```python
from build123d import *

# Parameters (mm, degrees)
SKETCH3_W                                      = 100
SKETCH3_H                                      = 100
BOSS_EXTRUDE2_DEPTH                            = 8
CBORE_FOR_2_SOCKET_HEAD_CAP_SCREW1_D           = 2.4384
CBORE_FOR_2_SOCKET_HEAD_CAP_SCREW1_CBORE_D     = 4.7625
CBORE_FOR_2_SOCKET_HEAD_CAP_SCREW1_CBORE_DEPTH = 2.1844
FILLET1_R                                      = 1
FILLET2_R                                      = 3
FILLET3_R                                      = 3


with BuildPart() as part:
    # Sketch3 → Boss-Extrude2 (new body)
    with BuildSketch(Plane(origin=(0, 0, 0), x_dir=(1, 0, 0), z_dir=(0, 1, 0))):
        Rectangle(SKETCH3_W, SKETCH3_H)
    extrude(amount=BOSS_EXTRUDE2_DEPTH)

    # CBORE for #2 Socket Head Cap Screw1 (through all)
    with Locations(Plane(origin=(-46, 8, 32), x_dir=(0, 0, 1), z_dir=(0, 1, 0))):
        with Locations((0, 0), (14, 14), (-64, 0), (-78, 14.320192801), (-78, 78), (-64, 92), (14, 78), (0, 92)):
            CounterBoreHole(CBORE_FOR_2_SOCKET_HEAD_CAP_SCREW1_D / 2, CBORE_FOR_2_SOCKET_HEAD_CAP_SCREW1_CBORE_D / 2, CBORE_FOR_2_SOCKET_HEAD_CAP_SCREW1_CBORE_DEPTH)

    # Fillet1
    fillet1_edges = [part.edges().sort_by_distance(p)[0] for p in [
        (-50, 8, 0),
        (0, 8, 50),
        (50, 8, 0),
        (0, 8, -50),
    ]]
    fillet(fillet1_edges, radius=FILLET1_R)

    # Fillet2
    # the kernel refuses this fillet: 3 mm, written as the material it takes off along each edge
    with BuildSketch(Plane(origin=(-47, 8, -47), x_dir=(0, 0, -1), z_dir=(1, 0, 0))) as fillet2_piece_1:
        with BuildLine():
            CenterArc((2, -1), 1, 0, 90)
            Line((3, -1), (3, 0))
            Line((3, 0), (2, 0))
        make_face()
    revolve(axis=Axis((-47, 8, -47), (0, 1, 0)), revolution_arc=90, mode=Mode.SUBTRACT)
    with BuildSketch(Plane(origin=(47, 8, -47), x_dir=(1, 0, 0), z_dir=(0, 0, 1))) as fillet2_piece_2:
        with BuildLine():
            CenterArc((2, -1), 1, 0, 90)
            Line((3, -1), (3, 0))
            Line((3, 0), (2, 0))
        make_face()
    revolve(axis=Axis((47, 8, -47), (0, 1, 0)), revolution_arc=90, mode=Mode.SUBTRACT)
    with BuildSketch(Plane(origin=(-47, 8, 47), x_dir=(-1, 0, 0), z_dir=(0, 0, -1))) as fillet2_piece_3:
        with BuildLine():
            CenterArc((2, -1), 1, 0, 90)
            Line((3, -1), (3, 0))
            Line((3, 0), (2, 0))
        make_face()
    revolve(axis=Axis((-47, 8, 47), (0, 1, 0)), revolution_arc=90, mode=Mode.SUBTRACT)
    with BuildSketch(Plane(origin=(-50, -7.5, 50), x_dir=(0, 0, -1), z_dir=(0, 1, 0)), Plane(origin=(-50, -7.5, -50), x_dir=(1, 0, 0), z_dir=(0, 1, 0))) as fillet2_piece_4:
        with BuildLine():
            CenterArc((FILLET2_R, -FILLET2_R), FILLET2_R, 90, 90)
            Line((0, -FILLET2_R), (0, 0))
            Line((0, 0), (FILLET2_R, 0))
        make_face()
    extrude(amount=15.5, mode=Mode.SUBTRACT)
    with BuildSketch(Plane(origin=(50, -7.5, -50), x_dir=(-1, 0, 0), z_dir=(0, 1, 0))) as fillet2_piece_5:
        with BuildLine():
            CenterArc((FILLET2_R, FILLET2_R), FILLET2_R, 180, 90)
            Line((0, FILLET2_R), (0, 0))
            Line((0, 0), (FILLET2_R, 0))
        make_face()
    extrude(amount=15.5, mode=Mode.SUBTRACT)

    # Fillet3
    # the kernel refuses this fillet: 3 mm, written as the material it takes off along each edge
    with BuildSketch(Plane(origin=(47, 8, 47), x_dir=(0, 0, 1), z_dir=(-1, 0, 0))) as fillet3_piece_1:
        with BuildLine():
            CenterArc((2, -1), 1, 0, 90)
            Line((3, -1), (3, 0))
            Line((3, 0), (2, 0))
        make_face()
    revolve(axis=Axis((47, 8, 47), (0, 1, 0)), revolution_arc=90, mode=Mode.SUBTRACT)
    with BuildSketch(Plane(origin=(50, -7.5, 50), x_dir=(-1, 0, 0), z_dir=(0, 1, 0))) as fillet3_piece_2:
        with BuildLine():
            CenterArc((FILLET3_R, -FILLET3_R), FILLET3_R, 90, 90)
            Line((0, -FILLET3_R), (0, 0))
            Line((0, 0), (FILLET3_R, 0))
        make_face()
    extrude(amount=15.5, mode=Mode.SUBTRACT)


solid = part.part
```
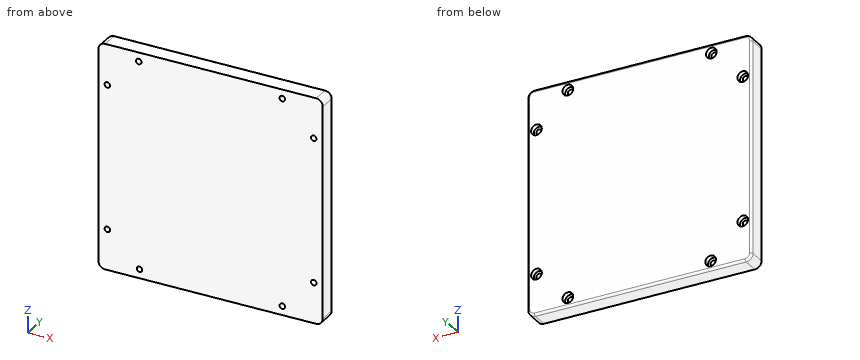
Here's how the part is built. I have some questions about the finished solid (model axes, mm). Coordinates: 2 decimals unless noted, no trailing zeros. Order: outer loops, then holes, each group sorted by start corner. A loop starts at its lowest first (then second) coordinate and runs counter-clockwise, first axis right, second up. Notation, with made-up numbers: M -22.75,51.25 L 6.25,51.25 A30 cw 6.25,82.25 Z; hole C -23.75,16.5 d1. An arc over 180 degrees is marked long. Answer as a JSON object with one key per item and string values. Group by question number.
(1) I need wall thicknesses on probe 1 along X at (y, z) = (6.95, -46); probe 2 along X at (y, z) = (7.4, 46); probe 3 along X at (y, z) = (7.5, -40). Which ranges of each line are inside material? Lowest first, please.
(2) Suppose I cut it at A-A, the plane z = 32. Please give me the cut outline in (x, y), then the cut area to 3 significant figures.
(3) For pin 1 (4 mm diameter, centred on x = 32, z = 46, fed in from +Y); pin 2 (10 mm diameter, centred on x = 13.5, z = 26, fed in from -Y); pin 3 (1.5 mm diameter, centred on x = -32, z = 46, fed in from -Y), each with a flat end and sliding along its axis, tell me the tip position at first contact or that it passes through.
Values found:
{
 "1": {"probe 1": "x = -50 to -34.06, -29.3 to 29.62, 34.38 to 50", "probe 2": "x = -49.92 to -34.38, -29.62 to 29.62, 34.38 to 49.92", "probe 3": "x = -49.87 to 49.87"},
 "2": {"outline": "M -50,0 L -47.22,0 L -47.22,5.82 L -48.38,5.82 L -48.38,8 L -49,8 A1 ccw -50,7 Z; M -44.78,0 L 44.78,0 L 44.78,5.82 L 43.62,5.82 L 43.62,8 L -43.62,8 L -43.62,5.82 L -44.78,5.82 Z; M 47.22,0 L 50,0 L 50,7 A1 ccw 49,8 L 48.38,8 L 48.38,5.82 L 47.22,5.82 Z", "area": "750 mm^2"},
 "3": {"pin 1": "stops at y = 5.82", "pin 2": "stops at y = 0", "pin 3": "passes through"}
}
